```python
from build123d import *

# Parameters (mm, degrees)
SKETCH1_R           = 20
SKETCH1_R_2         = 4
BOSS_EXTRUDE1_DEPTH = 10
SKETCH2_R           = 12.5
CUT_EXTRUDE1_DEPTH  = 3
FILLET1_R           = 2


with BuildPart() as part:
    # Sketch1 → Boss-Extrude1 (new body)
    with BuildSketch(Plane.XY):
        Circle(SKETCH1_R)
        Circle(SKETCH1_R_2, mode=Mode.SUBTRACT)
    extrude(amount=BOSS_EXTRUDE1_DEPTH)

    # Sketch2 → Cut-Extrude1 (cut)
    with BuildSketch(Plane.XY.offset(10)):
        Circle(SKETCH2_R)
    extrude(amount=-CUT_EXTRUDE1_DEPTH, mode=Mode.SUBTRACT)

    # Fillet1
    fillet1_edges = [part.edges().sort_by_distance(p)[0] for p in [
        (-20, 0, 0),
        (-20, 0, 10),
    ]]
    fillet(fillet1_edges, radius=FILLET1_R)


solid = part.part
```
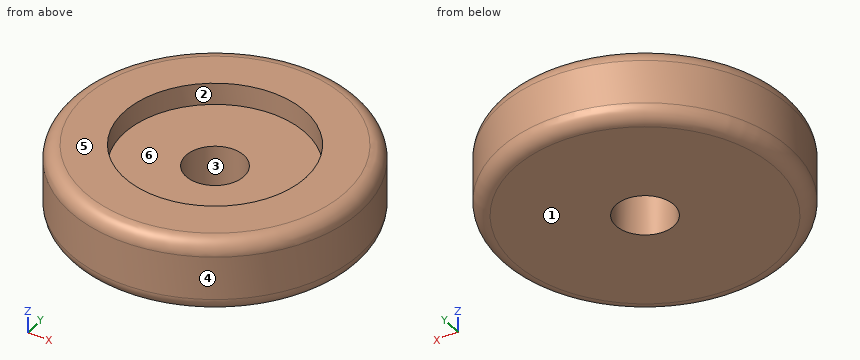
Source: CAD feature listing. Evaluate the final solid. Frame: model axes, mm. Face numbers are marked on the shaded views. A direction names the side the tool comes from. Coordinates: 2 decimals unless noted, no trailing zeros. Loops run counter-clockwise (first coordinate to the right, second up) from the corner with the lowest first, then second, coordinate; pieces in that order, holes last. Notation, with made-up numbers: M 8,59 L 34,59 A14 ccw 34,84 Z; hole C -17,-11 d4. An arc over 180 degrees is marked long. Use a Markdown table: item, result. Add a question column.
Q1. Access query for the marked faces 1 and 2. Directions: +Z, -Z, +X, -X, +Y, -Y. A direction counts if a zero-diameter tool reaches every point of the face in a straight line with its end or side. Return the directions, or none.
Q2. Section query D-D, the plane z = 1.5. Return loops of the section in (x, y).
Q3. Section query C-C, the plane z = 6.25. Return loops of the section in (x, y).
Q4. Section query A-A, the plane x = 0. Return loops of the section in (y, z), and give its area (3 significant figures).
Q5. Draft query along Y for the marked faces 3, 4, 5 and 6. Return one class per face: pulls with the +Y half, pulls with the -Y half, needs draft (parallel to the pull), parting line crosses it, or undercut.
Q6. First-contact query: pin 1 (2 mm diameter, centred on x = -3, y = -10, fed in from +Z); pin 2 (1 mm diameter, centred on x = 13, z = 7.5, fed in from +Y); pin 3 (1 mm diameter, centred on x = -14, z = 8.5, fed in from +Y). Flat tips, straight axial feed; report the tip coordinate or a pass-through.
Q7. Material intervals for L1, parallel to Y at x = 0, z = 5; L2, parallel to Z at x = 1.5, y = -5.5; L3, parallel to Y at x = -10, z = 7.5, sorted ascending.
Result:
| question | item | result |
|---|---|---|
| 1 | face 1 | -Z, +X, -X, +Y, -Y |
| 1 | face 2 | +Z |
| 2 | outline | C 0,0 d39.87; hole C 0,0 d8 |
| 3 | outline | C 0,0 d40; hole C 0,0 d8 |
| 4 | outline | M -20,2 A2 ccw -18,0 L -4,0 L -4,7 L -12.5,7 L -12.5,10 L -18,10 A2 ccw -20,8 Z; M 4,0 L 18,0 A2 ccw 20,2 L 20,8 A2 ccw 18,10 L 12.5,10 L 12.5,7 L 4,7 Z |
| 4 | area | 266 mm2 |
| 5 | face 3 | undercut |
| 5 | face 4 | parting line crosses it |
| 5 | face 5 | needs draft |
| 5 | face 6 | undercut |
| 6 | pin 1 | stops at z = 7 |
| 6 | pin 2 | stops at y = 15.61 |
| 6 | pin 3 | stops at y = 14.69 |
| 7 | L1 | y = -20 to -4, 4 to 20 |
| 7 | L2 | z = 0 to 7 |
| 7 | L3 | y = -17.32 to -7.5, 7.5 to 17.32 |
